Geometry check sheet. Reference: drawing and pictorial views, mm from the part's lowest x, y, z. A direction names the side the tool comes from. Round coordinates to 2 decimals unless told otherwise and drop trailing zeros. Loops run counter-clockwise (first coordinate to the right, second up) from the corner with the lowest first, then second, coordinate; pieces in that order, holes last. Notation, with made-up numbers: (80, 88) -> (111, 88) arc R18 ccw to (111, 111) -> close; hole circle Ø8 at (67.5, 0.5). An arc over 180 degrees is marked (long way). Use one line per item in the form item = value.
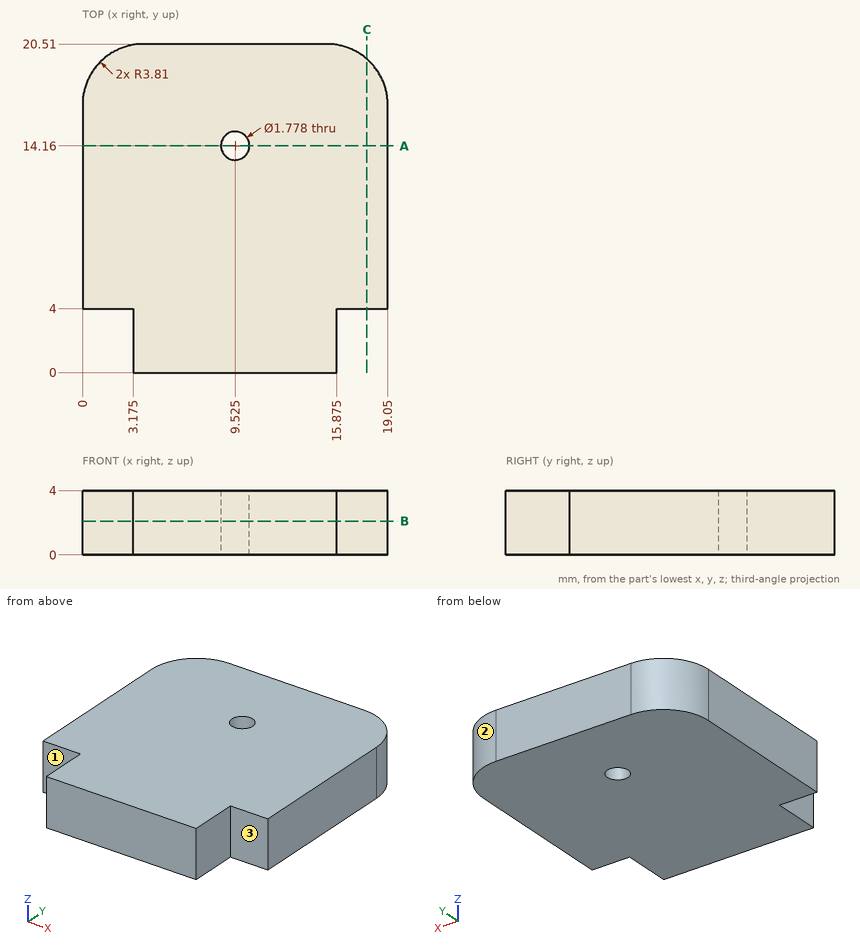
1. Material ranges on line 1 along X through (y, z) = (2.5, 0.65) (3 decimals); line 2 along Y through (x, z) = (9.25, 1.9); line 3 along Y through (x, z) = (8.75, 2.8), recorded low to high.
Return value:
line_1 = 3.175 to 15.875
line_2 = 0 to 13.31, 15.01 to 20.51
line_3 = 0 to 13.72, 14.6 to 20.51
2. Section check A-A (y = 14.16). Record the boundary of the cut face in (x, z).
Return value:
outline = (0, 0) -> (8.64, 0) -> (8.64, 4) -> (0, 4) -> close; (10.41, 0) -> (19.05, 0) -> (19.05, 4) -> (10.41, 4) -> close
3. Section check B-B (z = 2.1). Record the boundary of the cut face in (x, y) (3 decimals), then the cut area to 3 significant figures.
Return value:
outline = (0, 4) -> (3.175, 4) -> (3.175, 0) -> (15.875, 0) -> (15.875, 4) -> (19.05, 4) -> (19.05, 16.7) arc R3.81 ccw to (15.24, 20.51) -> (3.81, 20.51) arc R3.81 ccw to (0, 16.7) -> close; hole circle Ø1.778 at (9.525, 14.16)
area = 357 mm2
4. Section check C-C (x = 17.75). Record the boundary of the cut face in (y, z).
Return value:
outline = (4, 0) -> (19.57, 0) -> (19.57, 4) -> (4, 4) -> close
5. Tool access check on the marked faces 1, 2 and 3. Record the directions out of +Z, -Z, +X, -X, +Y, -Y that give a thin tool (end or side, any length) a straight path to the whole face; none if there is none.
Return value:
face_1 = +Z, -Z, -X, -Y
face_2 = +Z, -Z, +X, +Y
face_3 = +Z, -Z, +X, -Y
6. Gauge pin test, flat ends, axial feed: pin 1 (2 mm diameter, centred on y = 2.5, z = 1.5, fed in from -X) (3 decimals); pin 2 (1.6 mm diameter, centred on x = 1, z = 3, fed in from -Y). Record the tip position at first contact, or that the pin passes through.
Return value:
pin_1 = 3.175
pin_2 = 4
